from build123d import *

# Parameters (mm, degrees)
SKETCH1_R           = 1.5
SKETCH1_R_2         = 11.25
SKETCH1_R_3         = 2.1
SKETCH1_R_4         = 2.5
BOSS_EXTRUDE1_DEPTH = 2


with BuildPart() as part:
    # Sketch1 → Boss-Extrude1 (new body)
    with BuildSketch(Plane.XY):
        Polygon((0, 0), (20, 0), (20, -20), (105, -20), (105, 42), (0, 42), align=None)
        with Locations((3, 37)):
            Circle(SKETCH1_R, mode=Mode.SUBTRACT)
        with Locations((17, 37)):
            Circle(SKETCH1_R, mode=Mode.SUBTRACT)
        with Locations((84, 21)):
            Circle(SKETCH1_R_2, mode=Mode.SUBTRACT)
        with Locations((99.5, 36.5)):
            Circle(SKETCH1_R, mode=Mode.SUBTRACT)
        with Locations((68.5, 36.5)):
            Circle(SKETCH1_R, mode=Mode.SUBTRACT)
        with Locations((68.5, 5.5)):
            Circle(SKETCH1_R, mode=Mode.SUBTRACT)
        with Locations((99.5, 5.5)):
            Circle(SKETCH1_R, mode=Mode.SUBTRACT)
        with Locations((35, 32)):
            Circle(SKETCH1_R, mode=Mode.SUBTRACT)
        with Locations((28, 2)):
            Circle(SKETCH1_R, mode=Mode.SUBTRACT)
        with Locations((10, 28)):
            Circle(SKETCH1_R_3, mode=Mode.SUBTRACT)
        with Locations((10, 6)):
            Circle(SKETCH1_R_3, mode=Mode.SUBTRACT)
        with Locations((30, -10)):
            Circle(SKETCH1_R_3, mode=Mode.SUBTRACT)
        with Locations((95, -10)):
            Circle(SKETCH1_R_3, mode=Mode.SUBTRACT)
        with Locations((10, 37)):
            Circle(SKETCH1_R_4, mode=Mode.SUBTRACT)
        with Locations((50, -10)):
            Circle(SKETCH1_R_3, mode=Mode.SUBTRACT)
        with Locations((62, -10)):
            Circle(SKETCH1_R_3, mode=Mode.SUBTRACT)
    extrude(amount=BOSS_EXTRUDE1_DEPTH)


solid = part.part
Build history of the part. All positions in model axes, mm. A direction names the side the tool comes from. Coordinates: 2 decimals unless noted, no trailing zeros. Order: outer loops, then holes, each group sorted by start corner. A loop starts at its lowest first (then second) coordinate and runs counter-clockwise, first axis right, second up. Notation, with made-up numbers: (-30, 76.5) - (12, 76.5) arc R21 cw to (12, 112.5) - close; hole circle Ø5 at (36, 50.25). An arc over 180 degrees is marked (long way). Write item = value, one per line. Start each with the question number.
1) Saw through at D-D on z = 1.5. Count the separate pieces of the cut face and the enclosed holes in it, then the cut area to 3 significant figures.
2) Wall check: line 1 along Y through (x, z) = (68.5, 1.55); line 2 along Y through (x, z) = (30, 1.55); line 3 along Y through (x, z) = (80, 1.2). Give the ranges that are in metal, low to high. Write a range as from..to.
3) Saw through at B-B on x = 10. Write the cut outline in (y, z).
4) 3-axis set-ups, long thin cutter, end or side, ignore diameter. For faces 1 (the face through (10, 0, 1)), 2 (the face through (52, 11, 2)): which of +Z, -Z, +X, -X, +Y, -Y reach the whole face in a straight line?
5) Saw through at A-A on x = 84. Write the cut outline in (y, z), then the cut area to 3 significant figures.
6) Two-plate mould, pull along X, no slides. Class faces 3 (the face through (27.9, -9.91, 0.99)), 4 (the face through (105, 11, 1)), 5 (the face through (62, -20, 1)): pulls with the +X half, pulls with the -X half, needs draft (parallel to the pull), parting line crosses it, or undercut.
7) Saw through at C-C on y = 23. Write the cut outline in (x, z).
8) Flat gauge pin, fed straight in: pin 1 Ø2.5 at (x, y) = (62, -10) entering from +Z. Where does the tip first touch, or does it go through?
From the geometry:
q1.separate_pieces = 1
q1.enclosed_holes = 16
q1.area = 5,550 mm^2
q2.line_1 = -20..4, 7..35, 38..42
q2.line_2 = -20..-12.1, -7.9..42
q2.line_3 = -20..10.49, 31.51..42
q3.outline = (0, 0) - (3.9, 0) - (3.9, 2) - (0, 2) - close; (8.1, 0) - (25.9, 0) - (25.9, 2) - (8.1, 2) - close; (30.1, 0) - (34.5, 0) - (34.5, 2) - (30.1, 2) - close; (39.5, 0) - (42, 0) - (42, 2) - (39.5, 2) - close
q4.face_1 = +Z, -Z, -X, -Y
q4.face_2 = +Z, +X, -X, +Y, -Y
q5.outline = (-20, 0) - (9.75, 0) - (9.75, 2) - (-20, 2) - close; (32.25, 0) - (42, 0) - (42, 2) - (32.25, 2) - close
q5.area = 79.0 mm^2
q6.face_3 = undercut
q6.face_4 = pulls with the +X half
q6.face_5 = needs draft
q7.outline = (0, 0) - (72.93, 0) - (72.93, 2) - (0, 2) - close; (95.07, 0) - (105, 0) - (105, 2) - (95.07, 2) - close
q8.pin_1 = through
